Can you work these out from the model? Positions are in its coordinate system, mm. A direction names the side the tool comes from. Give positions to 0.01 mm unless a question says otherwise; leave off trailing zeros. Order: outer loops, then holes, each group sorted by start corner. A loop starts at its lowest first (then second) coordinate and runs counter-clockwise, first axis right, second up. Notation, with made-up numbers: (83.5, 3.5) -> (97.5, 3.5) arc R22 cw to (97.5, 12.5) -> close; hole circle Ø5 at (39.25, 44.25). An arc over 180 degrees is marked (long way). Answer as a JSON object with one key per item and string values.
```python
from build123d import *

# Parameters (mm, degrees)
F0_R     = 20
F1_DEPTH = 10
F2_T     = -3
F6_R     = 2.75
F7_DEPTH = 8
F9_D     = 3.5
F11_D    = 10
F13_D    = 10
F15_D    = 10
F17_D    = 10


# Not quite as in the source:
# - the program builds the solid bodies; features that only make, move or delete a surface that nothing else refers to are left out


with BuildPart() as f1:
    # F0 (on Top) → F1 (new body)
    with BuildSketch(Plane.XY):
        Circle(F0_R)
    extrude(amount=-F1_DEPTH)

    # F2
    f2_openings = [f1.faces().sort_by_distance(p)[0] for p in [
        (0, 0, 0),
    ]]
    offset(amount=F2_T, openings=f2_openings)

    # F6 (on face) → F7 (join)
    with BuildSketch(Plane.XY.offset(-7)):
        Circle(F6_R)
    extrude(amount=F7_DEPTH)

    # F9 (through all)
    with Locations(Plane.XY.offset(1)):
        with Locations((0, 0)):
            Hole(F9_D / 2)

    # F11 (through all)
    with Locations(Plane.XY):
        with Locations((-0.525876123, 10.7804676518)):
            Hole(F11_D / 2)

    # F13 (through all)
    with Locations(Plane.XY):
        with Locations((-9.7287148237, -0.5258764722)):
            Hole(F13_D / 2)

    # F15 (through all)
    with Locations(Plane.XY):
        with Locations((0.5258767051, -11.0434060916)):
            Hole(F15_D / 2)

    # F17 (through all)
    with Locations(Plane.XY):
        with Locations((11.3063445315, -0.7888147375)):
            Hole(F17_D / 2)


solid = f1.part
```
1. If we mould it in two halves opening along X, with no side actions, what happens to faces 1 (the face through (1.177, -6.086, -8.521)), 2 (the face through (-4.336, -19.524, -4.93)), 3 (the face through (0, -4, -10))? For each: +X half, -X half, draft (parallel to the pull), parting line (faces both ways), or undercut.
Worked answers:
{"face 1": "undercut", "face 2": "parting line", "face 3": "draft"}
2. If we section it at B-B on z = -6: Please give me the cut outline in (x, y).
Worked answers:
{"outline": "circle Ø40 at (0, 0); circle Ø5.5 at (0, 0); hole circle Ø34 at (0, 0); hole circle Ø3.5 at (0, 0)"}
3. Please list where these lines run through material, in increasing order: L1, parallel to Y at x = 0, z = -4.75; L2, parallel to Y at x = 3.5, z = -9; L3, parallel to X at y = 12, z = -4.25.
Worked answers:
{"L1": "-20 to -17, -2.75 to -1.75, 1.75 to 2.75, 17 to 20", "L2": "-19.69 to -15.06, -7.02 to 7.82, 13.75 to 19.69", "L3": "-16 to -12.04, 12.04 to 16"}
4. If we section it at C-C on y = 0: Please give me the cut outline in (x, z), then the cut area to 3 significant figures.
Worked answers:
{"outline": "(-20, -10) -> (-14.7, -10) -> (-14.7, -7) -> (-17, -7) -> (-17, 0) -> (-20, 0) -> close; (-4.76, -10) -> (-1.75, -10) -> (-1.75, 1) -> (-2.75, 1) -> (-2.75, -7) -> (-4.76, -7) -> close; (1.75, -10) -> (6.37, -10) -> (6.37, -7) -> (2.75, -7) -> (2.75, 1) -> (1.75, 1) -> close; (16.24, -10) -> (20, -10) -> (20, 0) -> (17, 0) -> (17, -7) -> (16.24, -7) -> close", "area": "108 mm²"}
5. Will these pins go through, and if not, where does the flat tip stop? pin 1 Ø8 at (x, y) = (0.53, -11.04) entering from +Z; pin 2 Ø4 at (y, z) = (5, -3.5) entering from -X; pin 3 Ø4 at (y, z) = (-9, -3) entering from -X (3 decimals); pin 4 Ø6 at (x, z) = (16, -7.5) entering from +Y.
Worked answers:
{"pin 1": "through", "pin 2": "x = -19.77", "pin 3": "x = -18.735", "pin 4": "y = 15.2"}
6. If we section it at A-A on x = 0: Please give me the cut outline in (y, z), then the cut area to 3 significant figures.
Worked answers:
{"outline": "(-20, -10) -> (-16.02, -10) -> (-16.02, -7) -> (-17, -7) -> (-17, 0) -> (-20, 0) -> close; (-6.07, -10) -> (-1.75, -10) -> (-1.75, 1) -> (-2.75, 1) -> (-2.75, -7) -> (-6.07, -7) -> close; (1.75, -10) -> (5.81, -10) -> (5.81, -7) -> (2.75, -7) -> (2.75, 1) -> (1.75, 1) -> close; (15.75, -10) -> (20, -10) -> (20, 0) -> (17, 0) -> (17, -7) -> (15.75, -7) -> close", "area": "108 mm²"}
7. For faces 4 (the face through (2, 0, 1)), 5 (the face through (-0.596, -2.685, -3.056)), which set-ups out of +Z, -Z, +X, -X, +Y, -Y let a thin tool reach every point of the face, with its end or its side?
Worked answers:
{"face 4": "+Z, +X, -X, +Y, -Y", "face 5": "+Z"}
8. If we section it at D-D on x = -14: Please give me the cut outline in (y, z), then the cut area to 3 significant figures.
Worked answers:
{"outline": "(-14.28, -10) -> (-3.13, -10) -> (-3.13, -7) -> (-9.64, -7) -> (-9.64, 0) -> (-14.28, 0) -> close; (2.07, -10) -> (14.28, -10) -> (14.28, 0) -> (9.64, 0) -> (9.64, -7) -> (2.07, -7) -> close", "area": "135 mm²"}
